Work out the finished part from the listing and answer in its coordinate system (mm). A direction names the side the tool comes from. Give positions to 0.01 mm unless a question says otherwise; leave off trailing zeros. Order: outer loops, then holes, each group sorted by start corner. A loop starts at its lowest first (then second) coordinate and runs counter-clockwise, first axis right, second up. Notation, with made-up numbers: (-13.5, 52) - (1.5, 52) arc R13 cw to (1.5, 61) - close; hole circle Ø5 at (62, 71). An arc over 180 degrees is marked (long way). Return JSON: item names as keys, results as strings. Group by question number.
from build123d import *

# Parameters (mm, degrees)
SALIENTE_EXTRUIR1_DEPTH = 25
CROQUIS2_R              = 2.5
CORTAR_EXTRUIR1_DEPTH   = 58.879184514


with BuildPart() as part:
    # Croquis1 → Saliente-Extruir1 (new body)
    with BuildSketch(Plane.XY):
        Polygon((15, 0), (0, 0), (0, 50), (15, 50), (15, 48), (2, 48), (2, 2), (15, 2), align=None)
    extrude(amount=SALIENTE_EXTRUIR1_DEPTH)

    # Croquis2 → Cortar-Extruir1 (cut, through all)
    with BuildSketch(Plane(origin=(0, 50, 0), x_dir=(1, 0, 0), z_dir=(0, 1, 0))):
        with Locations(Location((7.5, -12.5, 0), (0, 0, 270))):
            Circle(CROQUIS2_R)
    extrude(amount=-CORTAR_EXTRUIR1_DEPTH, mode=Mode.SUBTRACT)


solid = part.part
1. Determine the mould class of faces 3 (the flat face through (2, 25, 12)), 4 (the cylindrical face through (6, 49, 10.5)), 5 (the flat face through (1, 23, 25)) for opening direction X: released by +X, released by -X, zero draft, split by the parting line, or undercut.
2. A tool of negligible diameter and unlimited length cuts with its end or side. For faces 1 (the flat face through (15, 1, 12)), 2 (the flat face through (9, 48, 10)), from which of +Z, -Z, +X, -X, +Y, -Y can it reach the whole face along a straight path? Write none if from no direction.
3. The part is cut by section A-A (x = 11). Give the vertices of the cut face in (y, z).
4. This flat-tipped pin is pushed along its axis until it touches: pin 1 (5 mm diameter, centred on y = 31, z = 13, fed in from +X). Where does it stop, or does it pass through?
5. The part is cut by section B-B (z = 12.5). Give the vertices of the cut face in (x, y), and give its area (3 significant figures).
6. The part is cut by section C-C (x = 7.5). Give the vertices of the cut face in (y, z), and give its area (3 significant figures).
7. The part is cut by section D-D (z = 6.75). Give the vertices of the cut face in (x, y), and give its area (3 significant figures).
8. Consider probe 1 along Y at (x, z) = (5.75, 14.75); probe 2 along X at (y, z) = (0.55, 12.5); probe 3 along X at (y, z) = (21, 23.75). Determine where each line is inside the solid, lowest interval first. Write a range as from..to.
Answers:
{
 "1": {"face 3": "released by +X", "face 4": "undercut", "face 5": "zero draft"},
 "2": {"face 1": "+Z, -Z, +X, +Y, -Y", "face 2": "+Z, -Z, +X"},
 "3": {"outline": "(0, 0) - (2, 0) - (2, 25) - (0, 25) - close; (48, 0) - (50, 0) - (50, 25) - (48, 25) - close"},
 "4": {"pin 1": "stops at x = 2"},
 "5": {"outline": "(0, 0) - (5, 0) - (5, 2) - (2, 2) - (2, 48) - (5, 48) - (5, 50) - (0, 50) - close; (10, 0) - (15, 0) - (15, 2) - (10, 2) - close; (10, 48) - (15, 48) - (15, 50) - (10, 50) - close", "area": "132 mm^2"},
 "6": {"outline": "(0, 0) - (2, 0) - (2, 10) - (0, 10) - close; (0, 15) - (2, 15) - (2, 25) - (0, 25) - close; (48, 0) - (50, 0) - (50, 10) - (48, 10) - close; (48, 15) - (50, 15) - (50, 25) - (48, 25) - close", "area": "80.0 mm^2"},
 "7": {"outline": "(0, 0) - (15, 0) - (15, 2) - (2, 2) - (2, 48) - (15, 48) - (15, 50) - (0, 50) - close", "area": "152 mm^2"},
 "8": {"probe 1": "y = 0..2, 48..50", "probe 2": "x = 0..5, 10..15", "probe 3": "x = 0..2"}
}
